Drawing for the job (mm, zero at the part's lowest x, y, z). A direction names the side the tool comes from. Coordinates: 2 decimals unless noted, no trailing zeros. Write each loop counter-clockwise with the first axis right and the second up, starting at its lowest first coordinate (ties: lowest second). Pieces come first, ordered by that corner, then holes. Notation, with made-up numbers: (19, 31.25) -> (46, 31.25) arc R21 ccw to (46, 48.25) -> close; hole circle Ø4 at (-6, -2.5). An arc over 180 degrees is marked (long way). Answer as CSV lines item,"result". Start each with the question number.
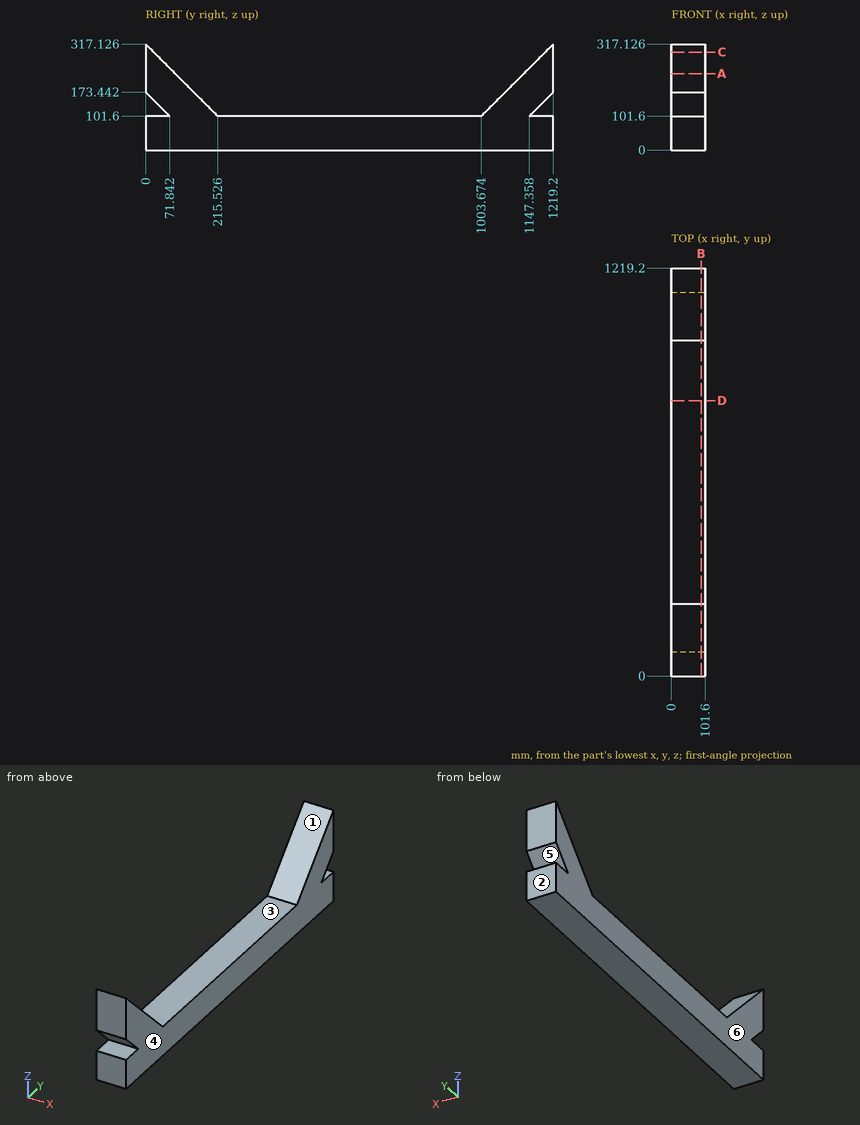
1. Cut at B-B (x = 89). Give the cut face in (y, z).
2. Mould opens along Y. For the marked faces 1, 2, 3 and 4 say: pulls with the +Y half, pulls with the -Y half, needs draft (parallel to the pull), parting line crosses it, or undercut.
3. Wall check: line 1 (Z direction, x = 52, y = 790.5); line 2 (Y direction, x = 80, z = 292); line 3 (Y direction, x = 22.5, z = 158). Give the ranges that are in metal, low to high.
4. Cut at A-A (z = 228.5). Give the cut face in (x, y).
5. Flat gauge pins, fed straight in: P1, Ø3, axis at x = 64.5, z = 66.5, coming from the -Y side; P2, Ø1.5, axis at x = 34.5, y = 604.5, coming from the +Z side; P3, Ø21.5, axis at x = 72, y = 1191.5, coming from the +Z side. Where does each tip first touch, or does it go through?
6. Cut at C-C (z = 293). Give the cut face in (x, y), then the cut area to 3 significant figures.
7. Tool access for the marked faces 5 and 6: list every direction of +Z, -Z, +X, -X, +Y, -Y with a clear straight run to the whole face (end or side of a thin tool).
8. Cut at D-D (y = 823). Give the cut face in (x, z), then the cut area to 3 significant figures.
Geometry check:
1,outline,"(0, 0) -> (1219.2, 0) -> (1219.2, 101.6) -> (1147.36, 101.6) -> (1219.2, 173.44) -> (1219.2, 317.13) -> (1003.67, 101.6) -> (215.53, 101.6) -> (0, 317.13) -> (0, 173.44) -> (71.84, 101.6) -> (0, 101.6) -> close"
2,face 1,"undercut"
2,face 2,"pulls with the +Y half"
2,face 3,"undercut"
2,face 4,"needs draft"
3,line 1,"0 to 101.6"
3,line 2,"0 to 25.13, 1194.07 to 1219.2"
3,line 3,"15.44 to 159.13, 1060.07 to 1203.76"
4,outline,"(0, 0) -> (101.6, 0) -> (101.6, 88.63) -> (0, 88.63) -> close; (0, 1130.57) -> (101.6, 1130.57) -> (101.6, 1219.2) -> (0, 1219.2) -> close"
5,P1,"y = 0"
5,P2,"z = 101.6"
5,P3,"z = 300.18"
6,outline,"(0, 0) -> (101.6, 0) -> (101.6, 24.13) -> (0, 24.13) -> close; (0, 1195.07) -> (101.6, 1195.07) -> (101.6, 1219.2) -> (0, 1219.2) -> close"
6,area,"4,900 mm²"
7,face 5,"+X, -X, +Y"
7,face 6,"+Z, -Z, -X, +Y, -Y"
8,outline,"(0, 0) -> (101.6, 0) -> (101.6, 101.6) -> (0, 101.6) -> close"
8,area,"10,300 mm²"
